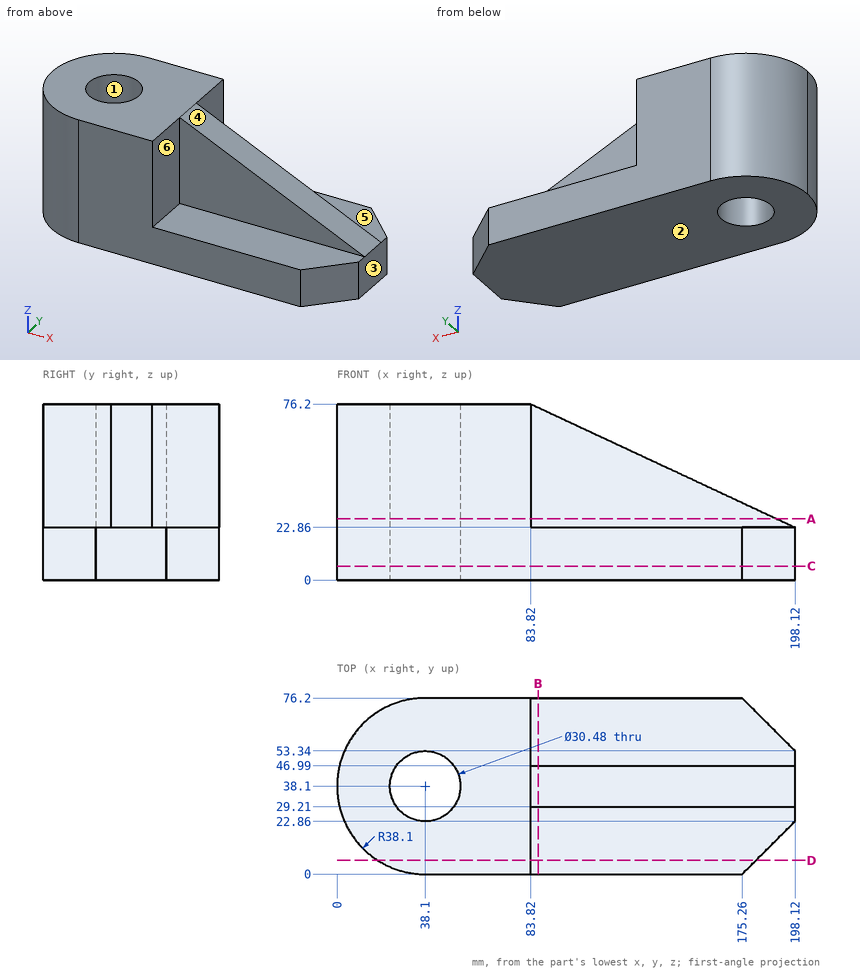
Input: dimensioned drawing with shaded views. Units: mm. Origin: part minimum x, y, z. A direction names the side the tool comes from. Coordinates: 2 decimals unless noted, no trailing zeros. Write each loop counter-clockwise with the first axis right and the second up, starting at its lowest first coordinate (ties: lowest second). Pieces come first, ordered by that corner, then holes. Notation, with made-up numbers: M 79.5,57 L 85.5,57 A16 cw 85.5,62 Z; hole C 57.25,35.25 d2. An arc over 180 degrees is marked long. Use a Markdown table: item, result.
1) Section D-D, the plane y = 6. Output: boundary loops of the cut face in (x, z).
Conclusion:
| item | result |
|---|---|
| outline | M 17.58,0 L 181.26,0 L 181.26,22.86 L 83.82,22.86 L 83.82,76.2 L 17.58,76.2 Z |
2) Ray query, L1, parallel to Y at x = 38.1, z = 19; L2, parallel to X at y = 35, z = 27.5; L3, parallel to X at y = 46.5, z = 15.5. Return the intervals inside material, ascending.
Conclusion:
| item | result |
|---|---|
| L1 | y = 0 to 22.86, 53.34 to 76.2 |
| L2 | x = 0.13 to 23.18, 53.02 to 188.18 |
| L3 | x = 0.94 to 25.38, 50.82 to 198.12 |
3) Section B-B, the plane x = 87. Output: boundary loops of the cut face in (y, z).
Conclusion:
| item | result |
|---|---|
| outline | M 0,0 L 76.2,0 L 76.2,22.86 L 46.99,22.86 L 46.99,74.72 L 29.21,74.72 L 29.21,22.86 L 0,22.86 Z |
4) First-contact query: pin 1 Ø2 at (x, y) = (176, 13.5) entering from +Z; pin 2 Ø14.5 at (y, z) = (66.5, 40.5) entering from +X; pin 3 Ø2 at (y, z) = (54.5, 22) entering from +X. Flat tips, straight axial feed; report the tip coordinate or a pass-through.
Conclusion:
| item | result |
|---|---|
| pin 1 | stops at z = 22.86 |
| pin 2 | stops at x = 83.82 |
| pin 3 | stops at x = 197.96 |
5) Mould query, pull axis X, two halves, no side actions, for the marked faces 1, 2 and 3. Classes: pulls with the +X half, pulls with the -X half, needs draft (parallel to the pull), parting line crosses it, or undercut.
Conclusion:
| item | result |
|---|---|
| face 1 | undercut |
| face 2 | needs draft |
| face 3 | pulls with the +X half |
6) Section A-A, the plane z = 26.5. Output: boundary loops of the cut face in (x, y), then the cut area to 3 significant figures.
Conclusion:
| item | result |
|---|---|
| outline | M 0,38.1 A38.1 ccw 38.1,0 L 83.82,0 L 83.82,29.21 L 190.32,29.21 L 190.32,46.99 L 83.82,46.99 L 83.82,76.2 L 38.1,76.2 A38.1 ccw Z; hole C 38.1,38.1 d30.48 |
| area | 6,930 mm^2 |
7) Section C-C, the plane z = 6. Output: boundary loops of the cut face in (x, y), then the cut area to 3 significant figures.
Conclusion:
| item | result |
|---|---|
| outline | M 0,38.1 A38.1 ccw 38.1,0 L 175.26,0 L 198.12,22.86 L 198.12,53.34 L 175.26,76.2 L 38.1,76.2 A38.1 ccw Z; hole C 38.1,38.1 d30.48 |
| area | 13,200 mm^2 |
8) Reachability of the marked faces 4, 5 and 6 from +Z, -Z, +X, -X, +Y, -Y: full face, straight path, thin tool, end or side. Return the list, or none.
Conclusion:
| item | result |
|---|---|
| face 4 | +Z, +X, +Y, -Y |
| face 5 | +Z, +X, +Y |
| face 6 | +Z, +X, -Y |
